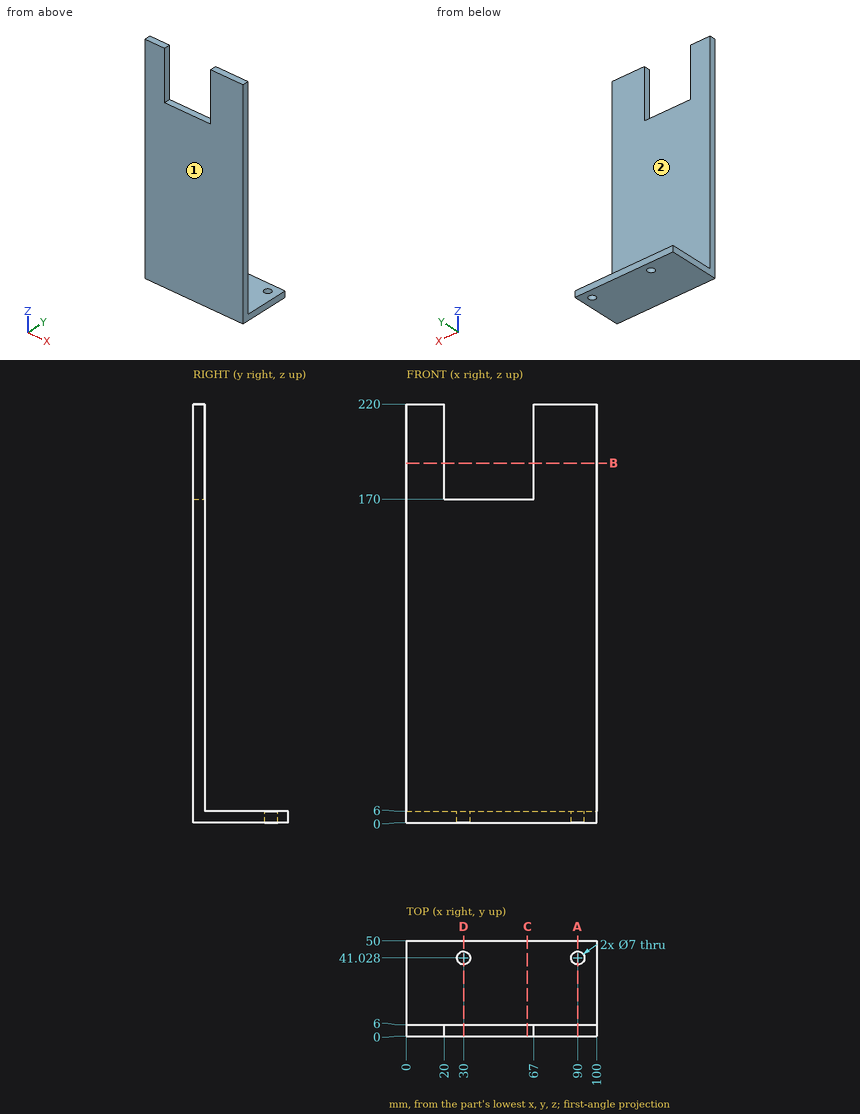
Input: dimensioned drawing with shaded views. Units: mm. Origin: part minimum x, y, z. A direction names the side the tool comes from. Coordinates: 2 decimals unless noted, no trailing zeros. Order: outer loops, then holes, each group sorted by start corner. A loop starts at its lowest first (then second) coordinate and runs counter-clockwise, first axis right, second up. Notation, with made-up numbers: M 31.25,-5.75 L 49.25,-5.75 A11 cw 49.25,4.25 Z; hole C -1.5,21 d7. An arc over 180 degrees is marked long. Answer as CSV lines item,"result".
Q1. Section C-C on x = 63.5. Return the cut outline in (y, z), and give its area (3 significant figures).
Answers:
outline,"M 0,0 L 50,0 L 50,6 L 6,6 L 6,170 L 0,170 Z"
area,"1,280 mm^2"
Q2. Section B-B on z = 189. Return the cut outline in (x, y).
Answers:
outline,"M 0,0 L 20,0 L 20,6 L 0,6 Z; M 67,0 L 100,0 L 100,6 L 67,6 Z"
Q3. First-contact query: P1, Ø6.5, axis at x = 30, y = 41.03, coming from the -Z side; P2, Ø8, axis at x = 45, y = 44.5, coming from the +Z side; P3, Ø6.5, axis at x = 35.5, y = 4.5, coming from the +Z side; P4, Ø1.8, axis at y = 3, z = 199.5, coming from the -X side. Flat tips, straight axial feed; report the tip coordinate or a pass-through.
Answers:
P1,"passes through"
P2,"stops at z = 6"
P3,"stops at z = 170"
P4,"stops at x = 0"
Q4. Section D-D on x = 30. Return the cut outline in (y, z).
Answers:
outline,"M 0,0 L 37.53,0 L 37.53,6 L 6,6 L 6,170 L 0,170 Z; M 44.53,0 L 50,0 L 50,6 L 44.53,6 Z"
Q5. Set-up query: the marked faces 1 and 2. Return all of +Z, -Z, +X, -X, +Y, -Y with unobstructed straight access to the full face (end or side cutting, diameter ignored); none if empty.
Answers:
face 1,"+Z, -Z, +X, -X, -Y"
face 2,"+Z, +X, -X, +Y"
Q6. Section A-A on x = 90. Return the cut outline in (y, z).
Answers:
outline,"M 0,0 L 37.53,0 L 37.53,6 L 6,6 L 6,220 L 0,220 Z; M 44.53,0 L 50,0 L 50,6 L 44.53,6 Z"
Q7. Line query: probe 1 along Y at (x, z) = (90, 4); probe 2 along Z at (x, y) = (45, 28); probe 3 along Z at (x, y) = (43, 3). Output: solid intervals per line, ascending. Write a range as [from, to].
Answers:
probe 1,"y = [0, 37.53], [44.53, 50]"
probe 2,"z = [0, 6]"
probe 3,"z = [0, 170]"
